CAD build for the part. Positions are in the model's coordinates, mm. A direction names the side the tool comes from. Give positions to 0.01 mm unless a question says otherwise; leave off trailing zeros. Write each loop counter-clockwise with the first axis right and the second up, starting at its lowest first coordinate (ties: lowest second). Pieces come first, ordered by that corner, then holes. Notation, with made-up numbers: (22, 86.5) - (40, 86.5) arc R28 ccw to (40, 115.5) - close; hole circle Ø6 at (22, 7.25). An arc over 180 degrees is marked (long way). Answer as a JSON object with one key per item and string values.
from build123d import *

# Parameters (mm, degrees)
SKIZZE1_W                       = 503
SKIZZE1_H                       = 107
AUFSATZ_LINEAR_AUSTRAGEN1_DEPTH = 350
SKIZZE2_R                       = 19
AUFSATZ_LINEAR_AUSTRAGEN2_DEPTH = 25


with BuildPart() as part:
    # Skizze1 → Aufsatz-Linear austragen1 (new body)
    with BuildSketch(Plane.XY):
        with Locations((251.5, 53.5)):
            Rectangle(SKIZZE1_W, SKIZZE1_H)
    extrude(amount=AUFSATZ_LINEAR_AUSTRAGEN1_DEPTH)

    # Skizze2 → Aufsatz-Linear austragen2 (add)
    with BuildSketch(Plane.XZ):
        with Locations(Location((84.399565915, 294.555551984, 0), (0, 0, 90))):
            Circle(SKIZZE2_R)
        with Locations(Location((403.747062166, 294.555551984, 0), (0, 0, 90))):
            Circle(SKIZZE2_R)
        with Locations(Location((403.747062166, 75.47123017, 0), (0, 0, 90))):
            Circle(SKIZZE2_R)
        with Locations(Location((84.399565915, 75.47123017, 0), (0, 0, 90))):
            Circle(SKIZZE2_R)
    extrude(amount=AUFSATZ_LINEAR_AUSTRAGEN2_DEPTH)


solid = part.part
(1) 3-axis set-ups, long thin cutter, end or side, ignore diameter. For faces 5 (the face through (422.295, -12.325, 71.352)), 6 (the face through (0, 53, 173)): which of +Z, -Z, +X, -X, +Y, -Y reach the whole face in a straight line?
Answer key:
{"face 5": "-Y", "face 6": "+Z, -Z, -X, +Y, -Y"}
(2) Saw through at A-A, the plane x = 49.5. Give the cut face in (y, z).
Answer key:
{"outline": "(0, 0) - (107, 0) - (107, 350) - (0, 350) - close"}
(3) Flat gauge pins, fed straight in: P1, Ø2, axis at y = 72.5, z = 289, coming from the -X side; P2, Ø6, axis at x = 326, z = 204.5, coming from the -Y side. Where does each tip first touch, or does it go through?
Answer key:
{"P1": "stops at x = 0", "P2": "stops at y = 0"}
(4) Pull direction Z, two halves, no side cores. Call faces 1 (the face through (101.256, -12.325, 84.239)), 2 (the face through (503, 53, 173)), 3 (the face through (415.31, -12.32, 279.48)), 4 (the face through (248, 54, 0)): pulls with the +Z half, pulls with the -Z half, needs draft (parallel to the pull), parting line crosses it, or undercut.
Answer key:
{"face 1": "undercut", "face 2": "needs draft", "face 3": "undercut", "face 4": "pulls with the -Z half"}
(5) Probe L1, parallel to Y at x = 296, z = 247; L2, parallel to Z at x = 77.5, y = -1. List the from-to ranges inside material, lowest first. Write a range as [from, to].
Answer key:
{"L1": "y = [0, 107]", "L2": "z = [57.77, 93.17], [276.85, 312.26]"}
(6) Saw through at B-B, the plane y = -13. Give the cut face in (x, z).
Answer key:
{"outline": "circle Ø38 at (84.4, 75.47); circle Ø38 at (84.4, 294.56); circle Ø38 at (403.75, 75.47); circle Ø38 at (403.75, 294.56)"}
(7) Saw through at C-C, the plane z = 190. Give the cut face in (x, y).
Answer key:
{"outline": "(0, 0) - (503, 0) - (503, 107) - (0, 107) - close"}
